For this review, take the finished solid that the model builds, in its own axes (mm). A direction names the side the tool comes from. Give positions to 0.01 mm unless a question says otherwise; leave off trailing zeros. Loops run counter-clockwise (first coordinate to the right, second up) from the corner with the lowest first, then second, coordinate; pieces in that order, holes last. Notation, with made-up numbers: (-19.75, -35.75) - (20.25, -35.75) arc R24 cw to (20.25, -23.75) - close; hole circle Ø5 at (67, -34). An arc over 180 degrees is marked (long way). Answer as CSV lines item,"result".
from build123d import *

# Parameters (mm, degrees)
SKETCH1_W           = 76.2
SKETCH1_H           = 38.1
SKETCH1_R           = 3.3274
BOSS_EXTRUDE1_DEPTH = 12.7
SKETCH5_R           = 3.175
BOSS_EXTRUDE3_DEPTH = 7.62
FILLET3_START       = -15.722599236
FILLET3_DEPTH       = 15.722599236
FILLET3_START_2     = -38.1
FILLET3_2_DEPTH     = 15.722595954
FILLET3_START_3     = -22.377404046
FILLET3_3_DEPTH     = 6.65480481
FILLET3_START_4     = 12.7
FILLET3_4_OUTLINE_R = 3.3274
FILLET3_4_DEPTH     = 20.32
SKETCH11_W          = 25.4
SKETCH11_H          = 19.05
CUT_EXTRUDE2_DEPTH  = 102.194377846
SKETCH13_R          = 6.35
CUT_EXTRUDE3_DEPTH  = 4.7625


with BuildPart() as part:
    # Sketch1 → Boss-Extrude1 (new body)
    with BuildSketch(Plane(origin=(0, 0, 0), x_dir=(1, 0, 0), z_dir=(0, 1, 0))):
        with Locations((38.1, 19.05)):
            Rectangle(SKETCH1_W, SKETCH1_H)
        with Locations(Location((19.05, 19.05, 0), (0, 0, 270))):
            Circle(SKETCH1_R, mode=Mode.SUBTRACT)
        with Locations(Location((57.15, 19.05, 0), (0, 0, 90))):
            Circle(SKETCH1_R, mode=Mode.SUBTRACT)
    extrude(amount=BOSS_EXTRUDE1_DEPTH)

    # Sketch5 → Boss-Extrude3 (add)
    with BuildSketch(Plane.ZY):
        with BuildLine():
            Line((-38.1, 12.7), (0, 12.7))
            Line((0, 12.7), (0, 48.26))
            ThreePointArc((0, 48.26), (-19.05, 67.31), (-38.1, 48.26))
            Line((-38.1, 48.26), (-38.1, 12.7))
        make_face()
        with Locations((-19.05, 48.26)):
            Circle(SKETCH5_R, mode=Mode.SUBTRACT)
    boss_extrude3 = extrude(amount=-BOSS_EXTRUDE3_DEPTH)

    # Fillet3: read off the stored shape, not the designer's step
    # Fillet3 outline → Fillet3 (add)
    with BuildSketch(Plane.XY.offset(FILLET3_START)):
        with BuildLine():
            Line((7.62, 12.7), (27.94, 12.7))
            ThreePointArc((27.94, 12.7), (13.571590206, 18.651590206), (7.62, 33.02))
            Line((7.62, 33.02), (7.62, 12.7))
        make_face()
    fillet3 = extrude(amount=FILLET3_DEPTH)

    # Fillet3 2 outline → Fillet3 2 (add)
    with BuildSketch(Plane.XY.offset(FILLET3_START_2)):
        with BuildLine():
            Line((7.62, 12.7), (27.94, 12.7))
            ThreePointArc((27.94, 12.7), (13.571590206, 18.651590206), (7.62, 33.02))
            Line((7.62, 33.02), (7.62, 12.7))
        make_face()
    fillet3_2 = extrude(amount=FILLET3_2_DEPTH)

    # Fillet3 3 outline → Fillet3 3 (add)
    with BuildSketch(Plane.XY.offset(FILLET3_START_3)):
        with BuildLine():
            Line((7.62, 12.7), (27.94, 12.7))
            ThreePointArc((27.94, 12.7), (13.571590206, 18.651590206), (7.62, 33.02))
            Line((7.62, 33.02), (7.62, 12.7))
        make_face()
    fillet3_3 = extrude(amount=FILLET3_3_DEPTH)

    # Fillet3 4 outline → Fillet3 4 (cut)
    with BuildSketch(Plane(origin=(0, 0, 0), x_dir=(1, 0, 0), z_dir=(0, 1, 0)).offset(FILLET3_START_4)):
        with Locations((19.05, 19.05)):
            Circle(FILLET3_4_OUTLINE_R)
    fillet3_4 = extrude(amount=FILLET3_4_DEPTH, mode=Mode.SUBTRACT)

    # Sketch11 → Cut-Extrude2 (cut, through all)
    with BuildSketch(Plane(origin=(0, 12.7, 0), x_dir=(1, 0, 0), z_dir=(0, 1, 0))):
        with Locations((20.32, 19.05)):
            Rectangle(SKETCH11_W, SKETCH11_H)
    cut_extrude2 = extrude(amount=CUT_EXTRUDE2_DEPTH, mode=Mode.SUBTRACT)

    # Sketch13 → Cut-Extrude3 (cut)
    with BuildSketch(Plane(origin=(7.62, 0, 0), x_dir=(0, 0, -1), z_dir=(1, 0, 0))):
        with Locations((19.05, 48.26)):
            Circle(SKETCH13_R)
    cut_extrude3 = extrude(amount=-CUT_EXTRUDE3_DEPTH, mode=Mode.SUBTRACT)

    # Mirror3: Boss-Extrude3, Fillet3, Fillet3 2, Fillet3 3, Fillet3 4 across plane
    add(boss_extrude3.mirror(Plane(origin=(38.1, 0, 0), x_dir=(0, 0, 1), z_dir=(1, 0, 0))))
    add(fillet3.mirror(Plane(origin=(38.1, 0, 0), x_dir=(0, 0, 1), z_dir=(1, 0, 0))))
    add(fillet3_2.mirror(Plane(origin=(38.1, 0, 0), x_dir=(0, 0, 1), z_dir=(1, 0, 0))))
    add(fillet3_3.mirror(Plane(origin=(38.1, 0, 0), x_dir=(0, 0, 1), z_dir=(1, 0, 0))))
    add(fillet3_4.mirror(Plane(origin=(38.1, 0, 0), x_dir=(0, 0, 1), z_dir=(1, 0, 0))), mode=Mode.SUBTRACT)

    # Mirror4: Cut-Extrude2 across plane
    add(cut_extrude2.mirror(Plane(origin=(38.1, 0, 0), x_dir=(0, 0, 1), z_dir=(1, 0, 0))), mode=Mode.SUBTRACT)

    # Mirror5: Cut-Extrude3 across plane
    add(cut_extrude3.mirror(Plane(origin=(38.1, 0, 0), x_dir=(0, 0, 1), z_dir=(1, 0, 0))), mode=Mode.SUBTRACT)


solid = part.part
1) Insertion check: P1, Ø3, axis at x = 33.5, z = -11.5, coming from the +Y side; P2, Ø8, axis at x = 17.5, z = -9, coming from the +Y side; P3, Ø5, axis at x = 22, z = -27, coming from the +Y side. Each pin has a flat end and moves straight along its axis. Give the tip position at first contact, or say it passes through.
From the geometry:
P1,"stops at y = 12.7"
P2,"stops at y = 18.72"
P3,"stops at y = 14.29"
2) Consider section B-B on y = 20. Write out the cut boundary in (x, z) (3 decimals), and give its area (3 significant figures).
From the geometry:
outline,"(0, -38.1) - (12.339, -38.1) - (12.339, -28.575) - (7.62, -28.575) - (7.62, -9.525) - (12.339, -9.525) - (12.339, 0) - (0, 0) - close; (63.861, -38.1) - (76.2, -38.1) - (76.2, 0) - (63.861, 0) - (63.861, -9.525) - (68.58, -9.525) - (68.58, -28.575) - (63.861, -28.575) - close"
area,"760 mm^2"
3) Consider section D-D on z = -4.5. Write out the cut boundary in (x, y).
From the geometry:
outline,"(0, 0) - (76.2, 0) - (76.2, 60.56) - (68.58, 60.56) - (68.58, 33.02) arc R20.32 cw to (48.26, 12.7) - (27.94, 12.7) arc R20.32 cw to (7.62, 33.02) - (7.62, 60.56) - (0, 60.56) - close"
4) Consider section A-A on z = -19.05. Count the separate pieces of the cut face and the enclosed holes in it, and give its area (3 significant figures).
From the geometry:
separate pieces,"5"
enclosed holes,"0"
area,"1,470 mm^2"
5) Consider section C-C on x = 57.15. Write out the cut boundary in (y, z) (3 decimals), and give its area (3 significant figures).
From the geometry:
outline,"(0, -38.1) - (14.748, -38.1) - (14.748, -28.575) - (12.7, -28.575) - (12.7, -22.377) - (0, -22.377) - close; (0, -15.723) - (12.7, -15.723) - (12.7, -9.525) - (14.748, -9.525) - (14.748, 0) - (0, 0) - close"
area,"438 mm^2"
6) Machinability: for faces 1 (the flat face through (0, 34, -19)), 2 (the flat face through (7.62, 40, -19)), 3 (the cylindrical face through (62.47, 18.494, -4.829)), 4 (the flat face through (76.2, 34, -19)), 5 (the flat face through (2.858, 50, -16)), which of the approach directions +Z, -Z, +X, -X, +Y, -Y give a long, thin tool a straight path to every point of the face, cutting with its end or side? Answer none if there is none.
From the geometry:
face 1,"+Z, -Z, -X, +Y, -Y"
face 2,"+Y"
face 3,"+Z, -Z, +Y"
face 4,"+Z, -Z, +X, +Y, -Y"
face 5,"none"
7) Wall thickness on line 1 (X direction, y = 8.5, z = -19.05); line 2 (X direction, y = 59.5, z = -12.5); line 3 (Z direction, x = 57, y = 7): over which ranges is each line inside the solid? List them lowest first. Write a range as from..to.
From the geometry:
line 1,"x = 0..15.72, 22.38..53.82, 60.48..76.2"
line 2,"x = 0..7.62, 68.58..76.2"
line 3,"z = -38.1..-22.37, -15.73..0"
8) Draft analysis for pull direction Z (two halves, no side actions). For faces 6 (the cylindrical face through (72.443, 67.305, -18.631)), 7 (the cylindrical face through (1.41, 51.41, -19.46)), 8 (the flat face through (38, 0, -19)), 9 (the flat face through (12, 18, -9.525)), state which applies: pulls with the +Z half, pulls with the -Z half, needs draft (parallel to the pull), parting line crosses it, or undercut.
From the geometry:
face 6,"parting line crosses it"
face 7,"undercut"
face 8,"needs draft"
face 9,"undercut"
